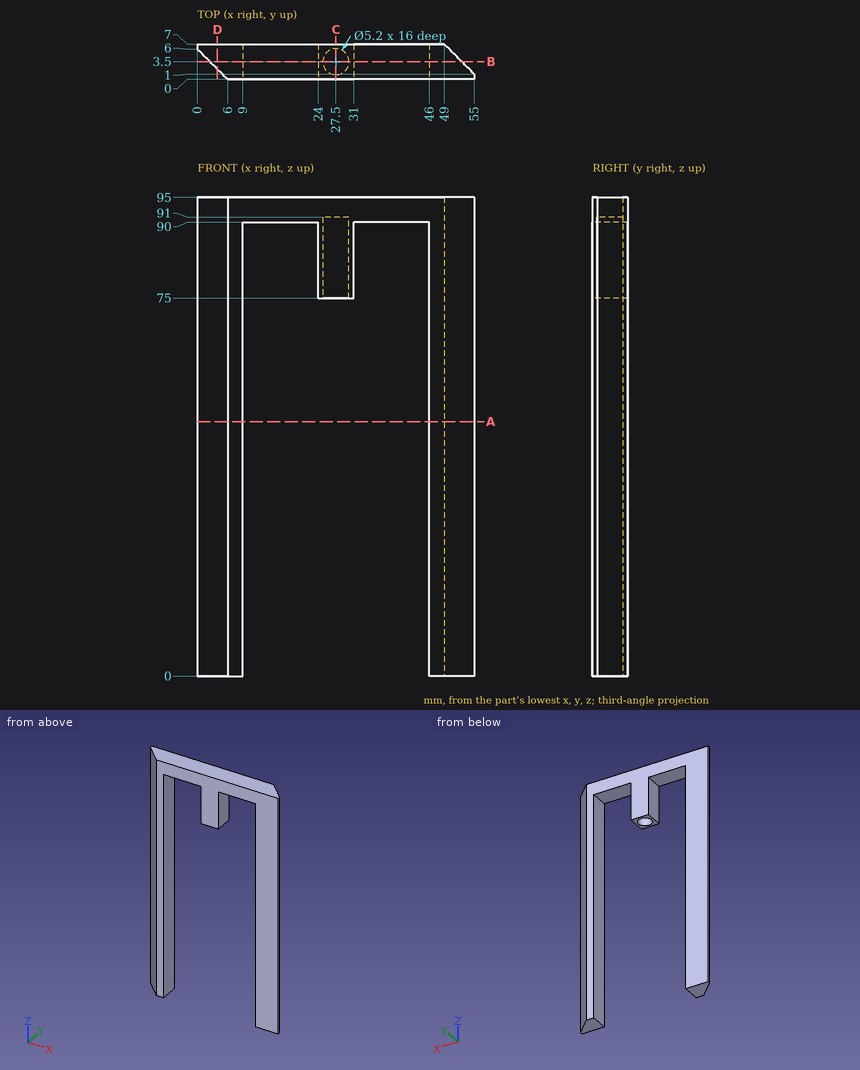
Part print with two shaded views. Sizes in mm from the minimum x, y, z corner. Round coordinates to 2 decimals unless told otherwise and drop trailing zeros. Loops run counter-clockwise (first coordinate to the right, second up) from the corner with the lowest first, then second, coordinate; pieces in that order, holes last. Notation, with made-up numbers: (76, -35.75) - (130, -35.75) arc R26 cw to (130, -1.75) - close; hole circle Ø7 at (40, 38). An arc over 180 degrees is marked (long way). Put each result on its own line as item: value.
1. Slice it at A-A on z = 50.5. List the corners of the cut face in (x, y), and give its area (3 significant figures).
Geometry check:
outline: (0, 6) - (6, 0) - (9, 0) - (9, 7) - (0, 7) - close; (46, 0) - (55, 0) - (55, 1) - (49, 7) - (46, 7) - close
area: 90.0 mm²
2. Pin check, flat tips, straight feed: P1, Ø3.5, axis at y = 3, z = 32.5, coming from the -X side; P2, Ø1.5, axis at y = 3, z = 12.5, coming from the -X side; P3, Ø3.5, axis at y = 4, z = 79, coming from the -X side. Stop position of each tip, or through.
Geometry check:
P1: x = 1.25
P2: x = 2.25
P3: x = 0.25
3. Slice it at D-D on x = 4. List the corners of the cut face in (y, z).
Geometry check:
outline: (2, 0) - (7, 0) - (7, 95) - (2, 95) - close
4. Slice it at C-C on x = 27.5. List the corners of the cut face in (y, z).
Geometry check:
outline: (0, 75) - (0.9, 75) - (0.9, 91) - (6.1, 91) - (6.1, 75) - (7, 75) - (7, 95) - (0, 95) - close
5. Slice it at B-B on y = 3.5. List the corners of the cut face in (x, z).
Geometry check:
outline: (2.5, 0) - (9, 0) - (9, 90) - (24, 90) - (24, 75) - (24.9, 75) - (24.9, 91) - (30.1, 91) - (30.1, 75) - (31, 75) - (31, 90) - (46, 90) - (46, 0) - (52.5, 0) - (52.5, 95) - (2.5, 95) - close
6. Wall check: line 1 (X direction, y = 1.25, z = 81); line 2 (Y direction, x = 27.5, z = 84.5); line 3 (Z direction, x = 45, y = 6.5). Give the ranges that are in metal, low to high.
Geometry check:
line 1: 4.75 to 9, 24 to 26.2, 28.8 to 31, 46 to 54.75
line 2: 0 to 0.9, 6.1 to 7
line 3: 90 to 95
